Verification items for the finished model (mm, model axes). A direction names the side the tool comes from. Round coordinates to 2 decimals unless told otherwise and drop trailing zeros. Return JSON: item names as keys, results as strings. Group by question number.
Item 1: Access from +Z, -Z, +X, -X, +Y, -Y to the whole of each face (thin tool, end or side, straight path). Record for faces 1 (the cylindrical face through (-1.05, 6.27, 7.54)), 2 (the flat face through (-2, 6, 5)), 3 (the cylindrical face through (-0.07, 3.54, -6.55)).
Item 2: Sectioned sample at A-A on x = 0. Give the number of separate pieces and of enclosed holes in the cut face, plus the area to 3 significant figures.
Item 3: Depth check by flat-ended pin: pin 1 Ø3.5 at (x, z) = (-1, 6) entering from -Y; pin 2 Ø1.4 at (x, z) = (-0.5, 5) entering from +Y; pin 3 Ø4 at (x, y) = (0, 4.5) entering from +Z; pin 4 Ø1 at (x, y) = (9.5, 5.5) entering from -Z. Enter the tip coordinate at first touch or a pass-through.
Item 4: Scan lines: probe 1 along X at (y, z) = (6.95, 5); probe 2 along X at (y, z) = (0.45, 0); probe 3 along Z at (x, y) = (-4, 6.5). Record each from-to range of solid material in increasing order. Write a range as from..to.
Item 5: Draft check along Z on faces 4 (the flat face through (0, 8, 0)), 5 (the cylindrical face through (13.856, 0.26, 5.745)), 6 (the flat face through (-2, 6, -5)). Enter one of: pulls with the +Z half, pulls with the -Z half, needs draft (parallel to the pull), parting line crosses it, or undercut.
```python
from build123d import *

# Parameters (mm, degrees)
CROQUIS6_R              = 14.5
CORTAR_EXTRUIR2_DEPTH   = 0.5
CROQUIS7_R              = 2.05
CROQUIS7_R_2            = 1.55
SALIENTE_EXTRUIR1_DEPTH = 6.5
CORTAR_EXTRUIR3_START   = -5.5
CROQUIS8_R              = 1.55
CORTAR_EXTRUIR3_DEPTH   = 5.5
REDONDEO1_R             = 2
REDONDEO2_R             = 2
CROQUIS9_R              = 2.75
CROQUIS9_R_2            = 1.55
SALIENTE_EXTRUIR2_DEPTH = 3
REDONDEO3_R             = 1
CROQUIS10_R             = 2.3
CORTAR_EXTRUIR6_DEPTH   = 2


with BuildPart() as part:
    # Croquis3 → Revolución1 (revolve)
    with BuildSketch(Plane.XY):
        with BuildLine():
            Line((15, 0), (15, 1.694213924))
            ThreePointArc((15, 1.694213924), (12.549846274, 2.962329925), (9.993557502, 4))
            ThreePointArc((9.993557502, 4), (9.70509179, 6.051742746), (9, 8))
            Line((9, 8), (0, 8))
            Line((0, 8), (0, 0))
            Line((0, 0), (15, 0))
        make_face()
    revolve(axis=Axis((0, 0, 0), (0, 1, 0)))

    # Croquis4 → Cortar-Revolución1 (revolve, cut)
    with BuildSketch(Plane.XY):
        with BuildLine():
            Line((0, 0.5), (0, 7.5))
            Line((0, 7.5), (8.680950348, 7.5))
            ThreePointArc((8.680950348, 7.5), (9.292895722, 5.613938885), (9.499999964, 3.641931911))
            ThreePointArc((9.499999964, 3.641931911), (12.052061122, 2.639235415), (14.5, 1.403916968))
            Line((14.5, 1.403916968), (14.5, 0.5))
            Line((14.5, 0.5), (0, 0.5))
        make_face()
    revolve(axis=Axis((0, 7.5, 0), (0, 1, 0)), mode=Mode.SUBTRACT)

    # Croquis6 → Cortar-Extruir2 (cut)
    with BuildSketch(Plane.XZ):
        Circle(CROQUIS6_R)
    extrude(amount=-CORTAR_EXTRUIR2_DEPTH, mode=Mode.SUBTRACT)

    # Croquis7 → Saliente-Extruir1 (add)
    # profile 1 of 2: a face of its own
    with BuildSketch(Plane.XZ.offset(-7.5)):
        with Locations(Location((0, 5, 0), (0, 0, 90))):
            Circle(CROQUIS7_R)
        with Locations(Location((0, 5, 0), (0, 0, 90))):
            Circle(CROQUIS7_R_2, mode=Mode.SUBTRACT)
    # profile 2 of 2: a face of its own
    with BuildSketch(Plane.XZ.offset(-7.5)):
        with Locations(Location((0, -5, 0), (0, 0, 90))):
            Circle(CROQUIS7_R)
        with Locations(Location((0, -5, 0), (0, 0, 90))):
            Circle(CROQUIS7_R_2, mode=Mode.SUBTRACT)
    extrude(amount=SALIENTE_EXTRUIR1_DEPTH)

    # Croquis8 → Cortar-Extruir3 (cut)
    with BuildSketch(Plane.XZ.offset(-7.5).offset(CORTAR_EXTRUIR3_START)):
        with Locations(Location((0, -5, 0), (0, 0, 90))):
            Circle(CROQUIS8_R)
        with Locations(Location((0, 5, 0), (0, 0, 90))):
            Circle(CROQUIS8_R)
    extrude(amount=CORTAR_EXTRUIR3_DEPTH, mode=Mode.SUBTRACT)

    # Redondeo1
    redondeo1_edges = [part.edges().sort_by_distance(p)[0] for p in [
        (-9, 8, 0),
    ]]
    fillet(redondeo1_edges, radius=REDONDEO1_R)

    # Redondeo2
    redondeo2_edges = [part.edges().sort_by_distance(p)[0] for p in [
        (-15, 1.694213924, 0),
    ]]
    fillet(redondeo2_edges, radius=REDONDEO2_R)

    # Croquis9 → Saliente-Extruir2 (add)
    # profile 1 of 2: a face of its own
    with BuildSketch(Plane(origin=(0, 8, 0), x_dir=(1, 0, 0), z_dir=(0, 1, 0))):
        with Locations(Location((0, 5, 0), (0, 0, 270))):
            Circle(CROQUIS9_R)
        with Locations(Location((0, 5, 0), (0, 0, 270))):
            Circle(CROQUIS9_R_2, mode=Mode.SUBTRACT)
    # profile 2 of 2: a face of its own
    with BuildSketch(Plane(origin=(0, 8, 0), x_dir=(1, 0, 0), z_dir=(0, 1, 0))):
        with Locations(Location((0, -5, 0), (0, 0, 270))):
            Circle(CROQUIS9_R)
        with Locations(Location((0, -5, 0), (0, 0, 270))):
            Circle(CROQUIS9_R_2, mode=Mode.SUBTRACT)
    extrude(amount=-SALIENTE_EXTRUIR2_DEPTH)

    # Redondeo3
    # the kernel refuses this fillet: 1 mm, written as the material it adds along each edge
    with BuildSketch(Plane(origin=(0, 5, -5), x_dir=(0, 0, 1), z_dir=(-1, 0, 0))) as redondeo3_piece_1:
        with BuildLine():
            CenterArc((3.05, -0.953939201), REDONDEO3_R, 107.457603124, 72.542396876)
            Line((2.75, 0), (2.744, 0.019078784))
            ThreePointArc((2.744, 0.019078784), (2.4, 0.02), (2.05, 0.02))
            Line((2.05, 0.02), (2.03, 0))
            Line((2.03, 0), (2.03, -0.953939201))
            Line((2.03, -0.953939201), (2.05, -0.953939201))
        make_face()
    revolve(axis=Axis((0, 5, -5), (0, 1, 0)))
    with BuildSketch(Plane(origin=(0, 5, 5), x_dir=(0, 0, 1), z_dir=(-1, 0, 0))) as redondeo3_piece_2:
        with BuildLine():
            CenterArc((3.05, -0.953939201), REDONDEO3_R, 107.457603124, 72.542396876)
            Line((2.05, -0.953939201), (2.03, -0.953939201))
            Line((2.03, -0.953939201), (2.03, 0))
            Line((2.03, 0), (2.05, 0.02))
            ThreePointArc((2.05, 0.02), (2.4, 0.02), (2.744, 0.019078784))
            Line((2.744, 0.019078784), (2.75, 0))
        make_face()
    revolve(axis=Axis((0, 5, 5), (0, 1, 0)))

    # Croquis10 → Cortar-Extruir6 (cut)
    with BuildSketch(Plane(origin=(0, 8, 0), x_dir=(1, 0, 0), z_dir=(0, 1, 0))):
        with Locations(Location((0, 5, 0), (0, 0, 270))):
            Circle(CROQUIS10_R)
        with Locations(Location((0, -5, 0), (0, 0, 270))):
            Circle(CROQUIS10_R)
    extrude(amount=-CORTAR_EXTRUIR6_DEPTH, mode=Mode.SUBTRACT)


solid = part.part
```
Recorded:
{
 "1": {"face 1": "-Y", "face 2": "+Y", "face 3": "+Y, -Y"},
 "2": {"separate pieces": "3", "enclosed holes": "0", "area": "30.4 mm²"},
 "3": {"pin 1": "y = 1", "pin 2": "through", "pin 3": "z = 13.51", "pin 4": "z = -3.97"},
 "4": {"probe 1": "-7.96..-7.37, -2.75..-2.3, 2.3..2.75, 7.37..7.96", "probe 2": "-15..-14.5, 14.5..15", "probe 3": "-8.71..-8.13, 8.13..8.71"},
 "5": {"face 4": "needs draft", "face 5": "parting line crosses it", "face 6": "undercut"}
}
